from build123d import *

# Parameters (mm, degrees)
SKETCH1_R           = 5
SKETCH2_R           = 3.1
CUT_EXTRUDE1_DEPTH  = 15
SKETCH4_W           = 3.376388604
SKETCH4_H           = 1
BOSS_EXTRUDE1_DEPTH = 9
SKETCH5_R           = 3.1
CUT_EXTRUDE2_DEPTH  = 240


with BuildPart() as part:
    # Sweep1: sweep along a curve in space
    with BuildLine() as sweep1_path:
        Line((0, 0, 0), (0, 0, -20))
        Line((0, 0, -20), (0, -240, -20))
    # Sketch1 → Sweep1 (sweep)
    with BuildSketch(Plane.XY):
        Circle(SKETCH1_R)
    sweep(path=sweep1_path.line, transition=Transition.RIGHT)

    # Sketch2 → Cut-Extrude1 (cut)
    with BuildSketch(Plane.XY):
        Circle(SKETCH2_R)
    extrude(amount=-CUT_EXTRUDE1_DEPTH, mode=Mode.SUBTRACT)

    # Sketch4 → Boss-Extrude1 (add)
    with BuildSketch(Plane.XY.offset(-15)):
        with Locations((0, -3.1)):
            Rectangle(SKETCH4_W, SKETCH4_H)
    extrude(amount=BOSS_EXTRUDE1_DEPTH)

    # Sketch5 → Cut-Extrude2 (cut)
    with BuildSketch(Plane.XZ.offset(240)):
        with Locations(Location((0, -20, 0), (0, 0, 270))):
            Circle(SKETCH5_R)
    extrude(amount=-CUT_EXTRUDE2_DEPTH, mode=Mode.SUBTRACT)


solid = part.part
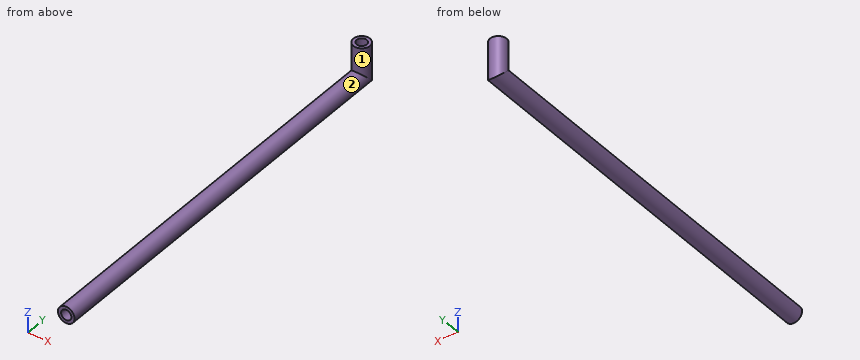
For this review, take the finished solid that the model builds, in its own axes (mm). Face numbers are marked on the shaded views. A direction names the side the tool comes from. Give positions to 0.01 mm unless a question says otherwise; leave off trailing zeros. Loops run counter-clockwise (first coordinate to the right, second up) from the corner with the lowest first, then second, coordinate; pieces in that order, holes last. Notation, with made-up numbers: M 55,77 L 73,77 A24 cw 73,89 Z; hole C 19.5,-2.5 d5. An arc over 180 degrees is marked long. Put each result on its own line as item: value. Start each with the question number.
(1) Machinability: for the marked faces 1 and 2, which of the approach directions +Z, -Z, +X, -X, +Y, -Y give a long, thin tool a straight path to every point of the face, cutting with its end or side? Answer none if there is none.
(2) Add section B-B, the plane y = -9.5. Write out the cut boundary in (x, z), then the cut area to 3 significant figures.
(3) Add section D-D, the plane z = -2.25. Write out the cut boundary in (x, y).
(4) Add section C-C, the plane x = 0. Write out the cut boundary in (y, z), then the cut area to 3 significant figures.
(5) Wall thickness on L1, parallel to Y at x = 0, z = -10; L2, parallel to X at y = 0, z = -3; L3, parallel to Z at x = -0.25, y = -96: over which ranges is each line inside the solid? List them lowest first.
(6) For pin 1 (3 mm diameter, centred on x = 1, z = -19.5, fed in from -Y); pin 2 (1 mm diameter, centred on x = -3.5, y = -171, fed in from -Z); pin 3 (2 mm diameter, centred on x = 3, z = -5.5, fed in from +Y), all flat-tipped, find the tip position at first contact; note any pin that passes through.
(7) Add section A-A, the plane z = -20. Write out the cut boundary in (x, y).
Result:
1. face 1: +Z
1. face 2: -Y
2. outline: C 0,-20 d10; hole C 0,-20 d6.2
2. area: 48.3 mm^2
3. outline: C 0,0 d10; hole C 0,0 d6.2
4. outline: M -240,-25 L 5,-25 L 5,0 L 3.1,0 L 3.1,-15 L -2.6,-15 L -2.6,-6 L -3.1,-6 L -3.1,0 L -5,0 L -5,-15 L -240,-15 L -240,-16.9 L 0,-16.9 L 0,-23.1 L -240,-23.1 Z
4. area: 1,020 mm^2
5. L1: y = -5 to -2.6, 3.1 to 5
5. L2: x = -5 to -3.1, 3.1 to 5
5. L3: z = -24.99 to -23.09, -16.91 to -15.01
6. pin 1: stops at y = 0
6. pin 2: stops at z = -24
6. pin 3: stops at y = 4.58
7. outline: M -5,-240 L -3.1,-240 L -3.1,0 L 3.1,0 L 3.1,-240 L 5,-240 L 5,0 A5 ccw -5,0 Z
